Verification items for the finished model (mm, model axes). Give positions to 0.01 mm unless a question says otherwise; leave off trailing zeros. Order: outer loops, then holes, each group sorted by start corner. A loop starts at its lowest first (then second) coordinate and runs counter-clockwise, first axis right, second up. Notation, with made-up numbers: M 28.5,-18.5 L 70.5,-18.5 A18 cw 70.5,8.5 Z; hole C 0.5,-7.5 d11. An arc over 180 degrees is marked long. Answer as a JSON object with one key per item and string values.
```python
from build123d import *

# Parameters (mm, degrees)
F0_W     = 457.2
F0_H     = 50.8
F1_DEPTH = 55.88
F2_R     = 4.445
F3_DEPTH = 111.76


with BuildPart() as f1:
    # F0 (on Front) → F1 (new body, symmetric)
    with BuildSketch(Plane.XZ):
        Rectangle(F0_W, F0_H)
    extrude(amount=F1_DEPTH, both=True)

    # F2 (on face) → F3 (cut, through all)
    with BuildSketch(Plane.XZ.offset(55.88)):
        with Locations((-128.559027, -5.007562)):
            Circle(F2_R)
        with Locations((23.840973, -5.007562)):
            Circle(F2_R)
        with Locations((176.240973, -5.007562)):
            Circle(F2_R)
    extrude(amount=-F3_DEPTH, mode=Mode.SUBTRACT)


solid = f1.part
```
Q1. Section check A-A on x = -128.5. Record the cut outline in (y, z), then the cut area to 3 significant figures.
Resolved:
{"outline": "M -55.88,-25.4 L 55.88,-25.4 L 55.88,-9.45 L -55.88,-9.45 Z; M -55.88,-0.56 L 55.88,-0.56 L 55.88,25.4 L -55.88,25.4 Z", "area": "4,680 mm²"}
Q2. Gauge pin test, flat end, axial feed: pin 1 Ø5.5 at (x, z) = (176.24, -5.01) entering from +Y. Record the tip position at first contact, or that the pin passes through.
Resolved:
{"pin 1": "passes through"}
Q3. Release check for a two-part mould opening along Z. For faces 1 (the face through (-3, 55.88, 0)), 2 (the face through (-3, -1, -25.4)), 3 (the face through (-3, -1, 25.4)), 4 (the face through (19.4, -0.8, -4.8)) record: +Z half, -Z half, draft (parallel to the pull), parting line (faces both ways), or undercut.
Resolved:
{"face 1": "draft", "face 2": "-Z half", "face 3": "+Z half", "face 4": "undercut"}
Q4. Material ranges on L1, parallel to X at y = 18.5, z = -5.5; L2, parallel to X at y = -34.5, z = -2, recorded low to high.
Resolved:
{"L1": "x = -228.6 to -132.98, -124.14 to 19.42, 28.26 to 171.82, 180.66 to 228.6", "L2": "x = -228.6 to -131.83, -125.29 to 20.57, 27.11 to 172.97, 179.51 to 228.6"}
